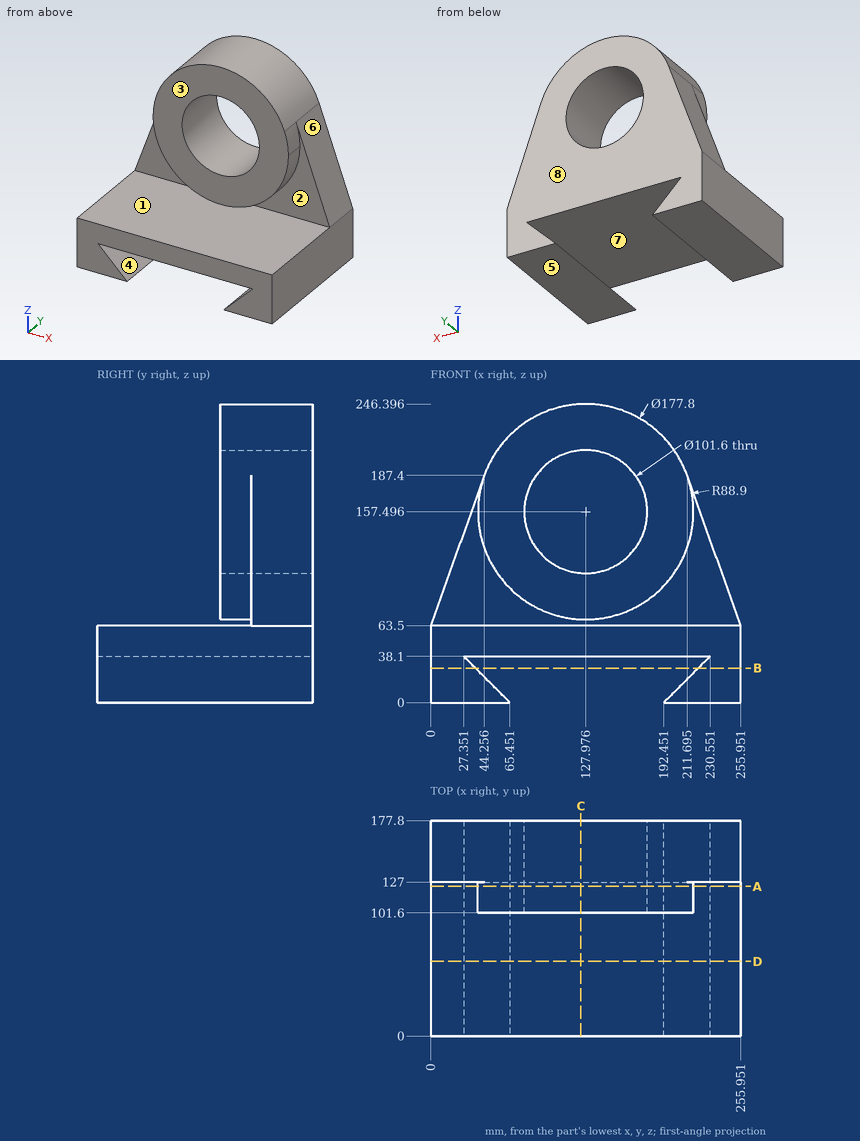
Can you work these out from the drawing? Everything is in mm from the part's minimum corner. A direction names the side the tool comes from. Give positions to 0.01 mm unless a question says otherwise; leave off trailing zeros. Order: outer loops, then holes, each group sorted by start corner. A loop starts at its lowest first (then second) coordinate and runs counter-clockwise, first axis right, second up. Notation, with made-up numbers: (23, 73) -> (80, 73) arc R19 ccw to (80, 83) -> close; hole circle Ø10 at (33, 20). An arc over 180 degrees is marked (long way). Return JSON: item names as keys, results as strings.
1. On a 3-axis mill with a long thin cutter (end or side, diameter ignored), from which of +Z, -Z, +X, -X, +Y, -Y can I reach the whole of each face in a straight line? I mean the marked faces 1, 2, 3, 4 and 5. Say none if no direction works.
Answer list:
{"face 1": "+X, -X, -Y", "face 2": "-Y", "face 3": "+Z, +X, -X, -Y", "face 4": "+Y, -Y", "face 5": "-Z, +X, -X, +Y, -Y"}
2. Imagine slicing it at A-A on y = 123.5. List the corners of the cut face in (x, z) for me (1 decimal), then the cut area to 3 significant figures.
Answer list:
{"outline": "(0, 0) -> (65.5, 0) -> (27.4, 38.1) -> (230.6, 38.1) -> (192.5, 0) -> (256, 0) -> (256, 63.5) -> (0, 63.5) -> close; (211.7, 187.4) arc R88.9 ccw (long way) to (216.9, 157.5) arc R88.9 ccw to start; hole circle Ø101.6 at (128, 157.5)", "area": "26,700 mm2"}
3. Imagine slicing it at C-C on x = 124. List the corners of the cut face in (y, z) for me (1 decimal), then the cut area to 3 significant figures.
Answer list:
{"outline": "(0, 38.1) -> (177.8, 38.1) -> (177.8, 106.9) -> (101.6, 106.9) -> (101.6, 68.7) -> (127, 68.7) -> (127, 63.5) -> (0, 63.5) -> close; (101.6, 208.1) -> (177.8, 208.1) -> (177.8, 246.3) -> (101.6, 246.3) -> close", "area": "10,600 mm2"}
4. Imagine slicing it at B-B on z = 28.5. List the corners of the cut face in (x, y) for me.
Answer list:
{"outline": "(0, 0) -> (36.95, 0) -> (36.95, 177.8) -> (0, 177.8) -> close; (220.95, 0) -> (255.95, 0) -> (255.95, 177.8) -> (220.95, 177.8) -> close"}
5. Thinking about a two-plate mould opening in X: for the marked faces 6, 7 and 8, which applies, pulls with the +X half, pulls with the -X half, needs draft (parallel to the pull), parting line crosses it, or undercut?
Answer list:
{"face 6": "pulls with the +X half", "face 7": "undercut", "face 8": "needs draft"}
6. I need wall thicknesses on line 1 (Z direction, x = 169, y = 108.5) (1 decimal); line 2 (Z direction, x = 142, y = 109); line 3 (Y direction, x = 102, z = 219.5). Which ranges of each line are inside material? Lowest first, please. Write a range as from..to.
Answer list:
{"line 1": "z = 38.1..63.5, 78.6..127.5, 187.5..236.4", "line 2": "z = 38.1..63.5, 69.71..108.67, 206.32..245.28", "line 3": "y = 101.6..177.8"}
7. For pin 1 Ø4 at (x, y) = (172.5, 104) entering from -Z; pin 2 Ø5 at (y, z) = (133.5, 77.5) entering from +X; pin 3 Ø6 at (y, z) = (119.5, 131.5) entering from +X, each with a flat end and sliding along its axis, tell me the tip position at first contact or that it passes through.
Answer list:
{"pin 1": "stops at z = 38.1", "pin 2": "stops at x = 251.84", "pin 3": "stops at x = 213.85"}
8. Imagine slicing it at D-D on y = 61.5. List the corners of the cut face in (x, z) for me.
Answer list:
{"outline": "(0, 0) -> (65.45, 0) -> (27.35, 38.1) -> (230.55, 38.1) -> (192.45, 0) -> (255.95, 0) -> (255.95, 63.5) -> (0, 63.5) -> close"}
